For this review, use the dimensioned drawing (mm, ordinates from the lowest corner) and the shaded views. A direction names the side the tool comes from. Round coordinates to 2 decimals unless told otherwise and drop trailing zeros. Write each loop counter-clockwise with the first axis right and the second up, starting at its lowest first coordinate (ties: lowest second). Pieces come first, ordered by that corner, then holes. Notation, with made-up numbers: M 35.5,-8 L 48.5,-8 A16 ccw 48.5,21 Z; hole C -31,73.25 d5. An arc over 180 degrees is marked long. Use one line per item in the form item = value. Start each with the question number.
Item 1: Draft analysis for pull direction X (two halves, no side actions). For the marked faces 3, 4 and 5, state which applies: released by +X, released by -X, zero draft, split by the parting line, or undercut.
Item 2: For line 1 (X direction, y = 0.6, z = 21.5); line 2 (Y direction, x = 24, z = 21); line 3 (Y direction, x = 13, z = 15), list the stretches that pass through material, from the lowest coordinate up. Write a range as [from, to].
Item 3: For P1, Ø3, axis at y = 33.5, z = 38, coming from the -X side; P2, Ø2, axis at y = 12, z = 30.5, coming from the -X side; P3, Ø1.5, axis at x = 25, y = 7, coming from the -Z side, all flat-tipped, find the tip position at first contact; note any pin that passes through.
Item 4: Add section C-C (y = 36.5). State the section outline as (x, z) points.
Item 5: For the marked faces 1 and 2, list the 3-axis set-ups (+Z, -Z, +X, -X, +Y, -Y) from which the entire face can be reached by the end or side of a thin tool; tool diameter is ignored.
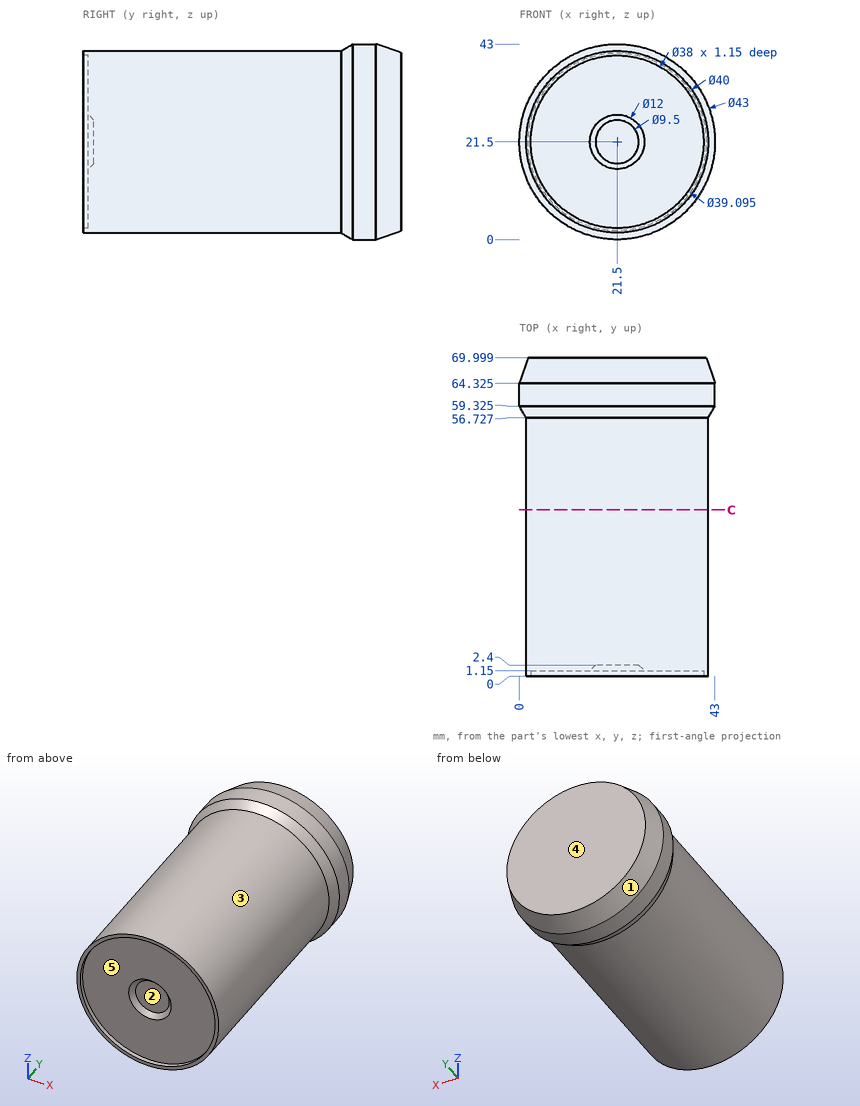
Calculated:
q1.face_3 = split by the parting line
q1.face_4 = zero draft
q1.face_5 = undercut
q2.line_1 = [1.5, 2.5], [40.5, 41.5]
q2.line_2 = [2.4, 70]
q2.line_3 = [1.15, 70]
q3.P1 = 8.27
q3.P2 = 3.17
q3.P3 = 1.69
q4.outline = C 21.5,21.5 d40
q5.face_1 = +Y
q5.face_2 = -Y
